```python
from build123d import *

# Parameters (mm, degrees)
SKETCH1_W           = 105.849999898
SKETCH1_H           = 152.4
BOSS_EXTRUDE1_DEPTH = 6.35
CUT_EXTRUDE1_REACH  = 94.994
SKETCH2_R           = 3.96875
SKETCH2_R_2         = 8.5


with BuildPart() as part:
    # Sketch1 → Boss-Extrude1 (new body)
    with BuildSketch(Plane(origin=(0, 0, 0), x_dir=(1, 0, 0), z_dir=(0, 1, 0))):
        Rectangle(SKETCH1_W, SKETCH1_H)
    extrude(amount=BOSS_EXTRUDE1_DEPTH)

    # Sketch2 → Cut-Extrude1 (cut, up to next)
    with BuildSketch(Plane(origin=(0, 6.35, 0), x_dir=(1, 0, 0), z_dir=(0, 1, 0)), mode=Mode.PRIVATE) as cut_extrude1_sk1:
        with Locations(Location((-27.524999949, -63.5, 0), (0, 0, 270))):
            Circle(SKETCH2_R)
    cut_extrude1_tool1 = extrude(cut_extrude1_sk1.sketch, amount=-CUT_EXTRUDE1_REACH, mode=Mode.PRIVATE) & part.part
    # Sketch2 → Cut-Extrude1 (cut, up to next)
    with BuildSketch(Plane(origin=(0, 6.35, 0), x_dir=(1, 0, 0), z_dir=(0, 1, 0)), mode=Mode.PRIVATE) as cut_extrude1_sk2:
        with Locations(Location((27.524999949, -63.5, 0), (0, 0, 270))):
            Circle(SKETCH2_R)
    cut_extrude1_tool2 = extrude(cut_extrude1_sk2.sketch, amount=-CUT_EXTRUDE1_REACH, mode=Mode.PRIVATE) & part.part
    # Sketch2 → Cut-Extrude1 (cut, up to next)
    with BuildSketch(Plane(origin=(0, 6.35, 0), x_dir=(1, 0, 0), z_dir=(0, 1, 0)), mode=Mode.PRIVATE) as cut_extrude1_sk3:
        with Locations(Location((-1.523999881, -28.34, 0), (0, 0, 270))):
            Circle(SKETCH2_R_2)
    cut_extrude1_tool3 = extrude(cut_extrude1_sk3.sketch, amount=-CUT_EXTRUDE1_REACH, mode=Mode.PRIVATE) & part.part
    add(cut_extrude1_tool1.solids().sort_by_distance((-27.525, 6.35, 63.5))[0], mode=Mode.SUBTRACT)
    add(cut_extrude1_tool2.solids().sort_by_distance((27.525, 6.35, 63.5))[0], mode=Mode.SUBTRACT)
    add(cut_extrude1_tool3.solids().sort_by_distance((-1.524, 6.35, 28.34))[0], mode=Mode.SUBTRACT)


solid = part.part
```
Geometry check sheet. Reference: the model listing, model coordinates, mm. Coordinates: 2 decimals unless noted, no trailing zeros. Order: outer loops, then holes, each group sorted by start corner. A loop starts at its lowest first (then second) coordinate and runs counter-clockwise, first axis right, second up. Notation, with made-up numbers: M 39,-6 L 76,-6 A25 cw 76,13 Z; hole C -20,29.25 d3. An arc over 180 degrees is marked long. Answer as a JSON object with one key per item and string values.
Q1. Cross-section at B-B on z = 63.5. Record the cut outline in (x, y) (3 decimals).
Results are:
{"outline": "M -52.925,0 L -31.494,0 L -31.494,6.35 L -52.925,6.35 Z; M -23.556,0 L 23.556,0 L 23.556,6.35 L -23.556,6.35 Z; M 31.494,0 L 52.925,0 L 52.925,6.35 L 31.494,6.35 Z"}
Q2. Cross-section at C-C on y = 4.5. Record the cut outline in (x, z) (1 decimal), and give its area (3 significant figures).
Results are:
{"outline": "M -52.9,-76.2 L 52.9,-76.2 L 52.9,76.2 L -52.9,76.2 Z; hole C -27.5,63.5 d7.9; hole C -1.5,28.3 d17; hole C 27.5,63.5 d7.9", "area": "15,800 mm²"}
Q3. Scan lines: line 1 (X direction, y = 3.5, z = 63.5) (3 decimals); line 2 (X direction, y = 2.5, z = 65.5) (3 decimals); line 3 (Z direction, x = -8, y = 3.5). Record each from-to range of solid material in increasing order.
Results are:
{"line 1": "x = -52.925 to -31.494, -23.556 to 23.556, 31.494 to 52.925", "line 2": "x = -52.925 to -30.953, -24.097 to 24.097, 30.953 to 52.925", "line 3": "z = -76.2 to 22.83, 33.85 to 76.2"}
Q4. Release check for a two-part mould opening along Z. For faces 1 (the flat face through (-1, 3, 76.2)), 2 (the cylindrical face through (1.029, 3.219, 36.447)), 3 (the flat face through (52.925, 3, 1)) record: released by +Z, released by -Z, zero draft, split by the parting line, or undercut.
Results are:
{"face 1": "released by +Z", "face 2": "undercut", "face 3": "zero draft"}
Q5. Cross-section at A-A on z = 28.34. Record the cut outline in (x, y) (3 decimals).
Results are:
{"outline": "M -52.925,0 L -10.024,0 L -10.024,6.35 L -52.925,6.35 Z; M 6.976,0 L 52.925,0 L 52.925,6.35 L 6.976,6.35 Z"}
